Build history of the part. All positions in model axes, mm. A direction names the side the tool comes from. Round coordinates to 2 decimals unless told otherwise and drop trailing zeros. Loops run counter-clockwise (first coordinate to the right, second up) from the corner with the lowest first, then second, coordinate; pieces in that order, holes last. Notation, with made-up numbers: M 27,60 L 50,60 A22 ccw 50,81 Z; hole C 65.5,-18.5 d6. An arc over 180 degrees is marked long. Use one line per item in the form item = value. Start each with the question number.
```python
from build123d import *

# Parameters (mm, degrees)
BOX030_W                   = 104
BOX030_H                   = 2.5
BOX030_DEPTH               = 40
BOX029_W                   = 107
BOX029_H                   = 3
BOX029_DEPTH               = 43
BOX028_W                   = 3
BOX028_H                   = 46
BOX028_DEPTH               = 2
CHAMFER003_SIZE            = 0.9
CHAMFER003_PLACEMENT_ANGLE = 90
BOX027_W                   = 3
BOX027_H                   = 46
BOX027_DEPTH               = 2
CHAMFER002_SIZE            = 0.9
CHAMFER002_PLACEMENT_ANGLE = 90
BOX031_W                   = 110
BOX031_H                   = 0.75
BOX031_DEPTH               = 46
FILLET_R                   = 1.5


with BuildPart() as cubo030:
    # Box030 → Box030 (new body)
    with BuildSketch(Plane(origin=(1.5, 27, 1.5), x_dir=(1, 0, 0), z_dir=(0, 0, 1))):
        with Locations((52, 1.25)):
            Rectangle(BOX030_W, BOX030_H)
    extrude(amount=BOX030_DEPTH)


with BuildPart() as cubo029:
    # Box029 → Box029 (new body)
    with BuildSketch(Plane(origin=(0, 27, 0), x_dir=(1, 0, 0), z_dir=(0, 0, 1))):
        with Locations((53.5, 1.5)):
            Rectangle(BOX029_W, BOX029_H)
    extrude(amount=BOX029_DEPTH)


with BuildPart() as chamfer003:
    # Box028 → Box028 (new body)
    with BuildSketch(Plane(origin=(5, -1, -6), x_dir=(1, 0, 0), z_dir=(0, 0, 1))):
        with Locations((1.5, 23)):
            Rectangle(BOX028_W, BOX028_H)
    extrude(amount=BOX028_DEPTH)

    # Chamfer003
    chamfer003_edges = [chamfer003.edges().sort_by_distance(p)[0] for p in [
        (6.5, -1, -6),
        (6.5, -1, -4),
        (6.5, 45, -6),
        (6.5, 45, -4),
    ]]
    chamfer(chamfer003_edges, length=CHAMFER003_SIZE)


with BuildPart() as chamfer003_1:
    # Chamfer003 placement: moved
    add(chamfer003.part.moved(Location((84, 23.7, -0.4))).rotate(Axis((84, 23.7, -0.4), (1, 0, 0)), CHAMFER003_PLACEMENT_ANGLE))


with BuildPart() as cut004:
    # Box027 → Box027 (new body)
    with BuildSketch(Plane(origin=(5, -1, -6), x_dir=(1, 0, 0), z_dir=(0, 0, 1))):
        with Locations((1.5, 23)):
            Rectangle(BOX027_W, BOX027_H)
    extrude(amount=BOX027_DEPTH)

    # Chamfer002
    chamfer002_edges = [cut004.edges().sort_by_distance(p)[0] for p in [
        (6.5, -1, -6),
        (6.5, -1, -4),
        (6.5, 45, -6),
        (6.5, 45, -4),
    ]]
    chamfer(chamfer002_edges, length=CHAMFER002_SIZE)


with BuildPart() as cut004_1:
    # Chamfer002 placement: moved
    add(cut004.part.moved(Location((12, 23.7, -0.4))).rotate(Axis((12, 23.7, -0.4), (1, 0, 0)), CHAMFER002_PLACEMENT_ANGLE))

    # Fusion001: union Chamfer003
    add(chamfer003_1.part)

    # Fusion002: union Cubo029
    add(cubo029.part)

    # Cut004: cut Cubo030
    add(cubo030.part, mode=Mode.SUBTRACT)


with BuildPart() as tapa:
    # Box031 → Box031 (new body)
    with BuildSketch(Plane(origin=(-1.5, 30, -1.5), x_dir=(1, 0, 0), z_dir=(0, 0, 1))):
        with Locations((55, 0.375)):
            Rectangle(BOX031_W, BOX031_H)
    extrude(amount=BOX031_DEPTH)

    # Fillet
    fillet_edges = [tapa.edges().sort_by_distance(p)[0] for p in [
        (-1.5, 30.375, 44.5),
        (-1.5, 30.375, -1.5),
        (108.5, 30.375, 44.5),
        (108.5, 30.375, -1.5),
    ]]
    fillet(fillet_edges, radius=FILLET_R)

    # Fusion003: union Cut004
    add(cut004_1.part)


solid = tapa.part
```
Q1. Tool access for faces 1 (the face through (105.5, 28, 21)), 2 (the face through (107, 28, 21)), 3 (the face through (0, 28, 21)), 4 (the face through (53, 30.75, 21)): list every direction of +Z, -Z, +X, -X, +Y, -Y with a clear straight run to the whole face (end or side of a thin tool).
Q2. Pull direction Z, two halves, no side cores. Call faces 5 (the face through (53, 28, 1.5)), 6 (the face through (53, 27, 42)), 7 (the face through (53, 29, 43)): pulls with the +Z half, pulls with the -Z half, needs draft (parallel to the pull), parting line crosses it, or undercut.
Q3. Saw through at B-B (x = 69). Give the cut face in (y, z).
Q4. Saw through at A-A (z = 22.5). Give the cut face in (x, y), and give its area (4 significant figures).
Q5. Wall check: probe 1 along X at (y, z) = (28.05, 10); probe 2 along Z at (x, y) = (79, 27.8); probe 3 along Y at (x, z) = (41, 15). Give the ranges that are in metal, low to high.
Q6. Drop flat-ended pins along their axis: P1, Ø2, axis at y = 27.5, z = 30, coming from the +X side; P2, Ø1.8, axis at y = 28.5, z = 43.5, coming from the -X side; P3, Ø20, axis at x = 63.5, z = 15.5, coming from the -Y side. Give the stop position or say it passes through.
Filled in:
q1.face_1 = -Y
q1.face_2 = +Z, -Z, +X, -Y
q1.face_3 = +Z, -Z, -X, -Y
q1.face_4 = +Z, -Z, +X, -X, +Y
q2.face_5 = undercut
q2.face_6 = needs draft
q2.face_7 = pulls with the +Z half
q3.outline = M 27,0 L 30,0 L 30,-1.5 L 30.75,-1.5 L 30.75,44.5 L 30,44.5 L 30,43 L 27,43 L 27,41.5 L 29.5,41.5 L 29.5,1.5 L 27,1.5 Z
q4.outline = M -1.5,30 L 0,30 L 0,27 L 1.5,27 L 1.5,29.5 L 105.5,29.5 L 105.5,27 L 107,27 L 107,30 L 108.5,30 L 108.5,30.75 L -1.5,30.75 Z
q4.area = 143.5 mm²
q5.probe_1 = 0 to 1.5, 105.5 to 107
q5.probe_2 = 0 to 1.5, 41.5 to 43
q5.probe_3 = 29.5 to 30.75
q6.P1 = 107
q6.P2 = 0
q6.P3 = 29.5
